Design review of the part built by this model. Coordinates are the model's own, in mm. Face numbers are marked on the shaded views. A direction names the side the tool comes from. Coordinates: 2 decimals unless noted, no trailing zeros. Write each loop counter-clockwise with the first axis right and the second up, starting at its lowest first coordinate (ties: lowest second). Pieces come first, ordered by that corner, then holes. Notation, with made-up numbers: (25, 32) -> (60, 32) arc R18 cw to (60, 59) -> close; hole circle Ø5 at (65.25, 12). An arc over 180 degrees is marked (long way). Answer in a Markdown table with one row per item. Add a question column.
Item 1: Take a section at A-A, the plane x = 7.5. Write out the cut boundary in (y, z), and give its area (3 significant figures).
Item 2: Take a section at C-C, the plane x = 2. Write out the cut boundary in (y, z), and give its area (3 significant figures).
Item 3: To check wall thickness, follow line 1 (Z direction, x = 2.5, y = 1); line 2 (X direction, y = -1, z = -5.5); line 3 (X direction, y = 2.75, z = 2). State the ranges of each line that lie inside material, in increasing order.
Item 4: For the marked faces 3, 4, 5, 6 and 7, list the 3-axis set-ups (+Z, -Z, +X, -X, +Y, -Y) from which the entire face can be reached by the end or side of a thin tool; tool diameter is ignored.
Item 5: Draft analysis for pull direction X (two halves, no side actions). For the marked faces 1 and 2, state which applies: released by +X, released by -X, zero draft, split by the parting line, or undercut.
Item 6: Take a section at B-B, the plane z = 6.75. Write out the cut boundary in (x, y).
Item 7: Clearance check with flat-ended pins moving along their axes: P1, Ø2, axis at x = 0, y = 0, coming from the +Z side; P2, Ø2, axis at x = -9, y = -1.5, coming from the +Z side; P3, Ø2.5, axis at x = -11, z = 5.5, coming from the +Y side. State where each tip first meets the part, or that it passes through.
Item 8: Take a section at D-D, the plane z = -5.75. Write out the cut boundary in (x, y), and give its area (3 significant figures).
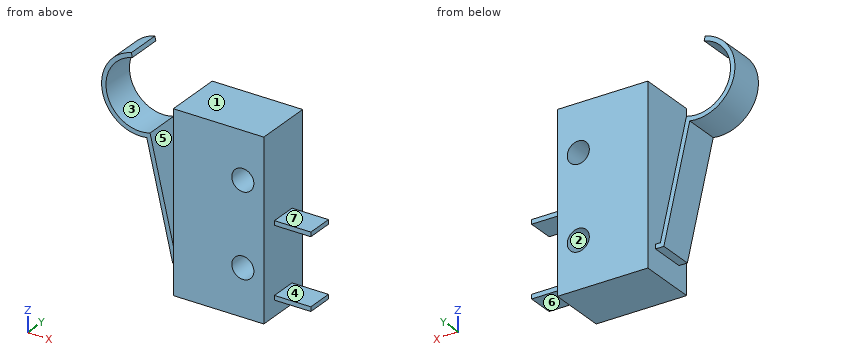
from build123d import *

# Parameters (mm, degrees)
SKETCH1_W           = 10.414
SKETCH1_H           = 20.32
SKETCH1_R           = 1.27
BOSS_EXTRUDE1_DEPTH = 3.3655
SKETCH1_3_W         = 4.191
SKETCH1_3_H         = 0.508
BOSS_EXTRUDE2_DEPTH = 1.524
BOSS_EXTRUDE3_DEPTH = 2.032


with BuildPart() as part:
    # Sketch1 → Boss-Extrude1 (new body, symmetric)
    with BuildSketch(Plane(origin=(0, 0, 0), x_dir=(1, 0, 0), z_dir=(0, 1, 0))):
        Rectangle(SKETCH1_W, SKETCH1_H)
        with Locations((2.794, -4.7625)):
            Circle(SKETCH1_R, mode=Mode.SUBTRACT)
        with Locations((2.794, 4.7625)):
            Circle(SKETCH1_R, mode=Mode.SUBTRACT)
    extrude(amount=BOSS_EXTRUDE1_DEPTH, both=True)

    # Sketch1_3 → Boss-Extrude2 (add, symmetric)
    with BuildSketch(Plane(origin=(0, 0, 0), x_dir=(1, 0, 0), z_dir=(0, 1, 0))):
        with Locations((7.3025, 0)):
            Rectangle(SKETCH1_3_W, SKETCH1_3_H)
        with Locations((7.3025, 8.128)):
            Rectangle(SKETCH1_3_W, SKETCH1_3_H)
    extrude(amount=BOSS_EXTRUDE2_DEPTH, both=True)

    # Sketch1_4 → Boss-Extrude3 (add, symmetric)
    with BuildSketch(Plane(origin=(0, 0, 0), x_dir=(1, 0, 0), z_dir=(0, 1, 0))):
        with BuildLine():
            Line((-5.207, 6.985), (-5.207, 7.493))
            Line((-5.207, 7.493), (-6.170558218, 7.493))
            Line((-6.170558218, 7.493), (-9.145014336, -5.25524689))
            ThreePointArc((-9.145014336, -5.25524689), (-14.261834387, -8.748771053), (-10.915992225, -13.963356246))
            Line((-10.915992225, -13.963356246), (-10.800564542, -13.468643754))
            ThreePointArc((-10.800564542, -13.468643754), (-13.709152444, -8.616780848), (-8.76594289, -5.866301519))
            Line((-8.76594289, -5.866301519), (-5.767441782, 6.985))
            Line((-5.767441782, 6.985), (-5.207, 6.985))
        make_face()
    extrude(amount=BOSS_EXTRUDE3_DEPTH, both=True)


solid = part.part
Answers:
| question | item | result |
|---|---|---|
| 1 | outline | (-1.52, -8.38) -> (1.52, -8.38) -> (1.52, -7.87) -> (-1.52, -7.87) -> close; (-1.52, -0.25) -> (1.52, -0.25) -> (1.52, 0.25) -> (-1.52, 0.25) -> close |
| 1 | area | 3.10 mm^2 |
| 2 | outline | (-3.37, -10.16) -> (3.37, -10.16) -> (3.37, -5.75) -> (-3.37, -5.75) -> close; (-3.37, -3.77) -> (3.37, -3.77) -> (3.37, 3.77) -> (-3.37, 3.77) -> close; (-3.37, 5.75) -> (3.37, 5.75) -> (3.37, 10.16) -> (-3.37, 10.16) -> close |
| 2 | area | 110 mm^2 |
| 3 | line 1 | z = -10.16 to -6, -3.53 to 3.53, 6 to 10.16 |
| 3 | line 2 | x = -6.64 to -6.11, -5.21 to 1.76, 3.83 to 5.21 |
| 3 | line 3 | x = -5.21 to 5.21 |
| 4 | face 3 | +Y, -Y |
| 4 | face 4 | +X, +Y, -Y |
| 4 | face 5 | +Z, +Y, -Y |
| 4 | face 6 | -Z, +X, +Y, -Y |
| 4 | face 7 | +Z, +X, +Y, -Y |
| 5 | face 1 | zero draft |
| 5 | face 2 | undercut |
| 6 | outline | (-13.29, -2.03) -> (-12.59, -2.03) -> (-12.59, 2.03) -> (-13.29, 2.03) -> close; (-5.21, -3.37) -> (5.21, -3.37) -> (5.21, 3.37) -> (-5.21, 3.37) -> close |
| 7 | P1 | stops at z = 10.16 |
| 7 | P2 | stops at z = 5.87 |
| 7 | P3 | stops at y = 2.03 |
| 8 | outline | (-6.58, -2.03) -> (-6.06, -2.03) -> (-6.06, 2.03) -> (-6.58, 2.03) -> close; (-5.21, -3.37) -> (2, -3.37) -> (2, 3.37) -> (-5.21, 3.37) -> close; (3.59, -3.37) -> (5.21, -3.37) -> (5.21, 3.37) -> (3.59, 3.37) -> close |
| 8 | area | 61.5 mm^2 |
